from build123d import *

# Parameters (mm, degrees)
SKETCH1_R           = 22.5
SKETCH1_R_2         = 11
BOSS_EXTRUDE1_DEPTH = 11.66


with BuildPart() as part:
    # Sketch1 → Boss-Extrude1 (new body)
    with BuildSketch(Plane(origin=(0, 0, 0), x_dir=(1, 0, 0), z_dir=(0, 1, 0))):
        Circle(SKETCH1_R)
        Circle(SKETCH1_R_2, mode=Mode.SUBTRACT)
    extrude(amount=BOSS_EXTRUDE1_DEPTH)

    # Sketch2 → Revolve1 (revolve)
    with BuildSketch(Plane.XY):
        Polygon((22.5, 11.66), (24.5, 11.66), (24.5, 10.66), (22.5, 10.33), align=None)
        Polygon((22.5, 0.33), (24.5, 0), (24.5, -1), (22.5, -1), (9, -1), (9, 0.33), (9, 4.66), (22.5, 4.66), align=None)
    revolve(axis=Axis((0, 0, 0), (0, 1, 0)))


solid = part.part
Verification items for the finished model (mm, model axes). A direction names the side the tool comes from. Coordinates: 2 decimals unless noted, no trailing zeros. Write each loop counter-clockwise with the first axis right and the second up, starting at its lowest first coordinate (ties: lowest second). Pieces come first, ordered by that corner, then holes. Notation, with made-up numbers: (85, 79.25) - (133, 79.25) arc R21 ccw to (133, 105.25) - close; hole circle Ø10 at (56, 60). An arc over 180 degrees is marked (long way). Answer as a JSON object with one key per item and string values.
(1) Cross-section at D-D on y = 5.5. Record the cut outline in (x, z).
Report:
{"outline": "circle Ø45 at (0, 0); hole circle Ø22 at (0, 0)"}
(2) Cross-section at B-B on z = 0. Record the cut outline in (x, y).
Report:
{"outline": "(-24.5, -1) - (-9, -1) - (-9, 4.66) - (-11, 4.66) - (-11, 11.66) - (-24.5, 11.66) - (-24.5, 10.66) - (-22.5, 10.33) - (-22.5, 0.33) - (-24.5, 0) - close; (9, -1) - (24.5, -1) - (24.5, 0) - (22.5, 0.33) - (22.5, 10.33) - (24.5, 10.66) - (24.5, 11.66) - (11, 11.66) - (11, 4.66) - (9, 4.66) - close"}
(3) Mould release check, pull along X, two halves, no side actions. Record for faces 3 (the flat face through (-2, 4.66, 9)), 4 (the cylindrical face through (10.382, 5.26, 19.961)), 5 (the flat face through (-11, -1, 0)): pulls with the +X half, pulls with the -X half, needs draft (parallel to the pull), parting line crosses it, or undercut.
Report:
{"face 3": "undercut", "face 4": "parting line crosses it", "face 5": "needs draft"}
(4) Tool access check on faces 1 (the cylindrical face through (-2.38, 8.11, 10.74)), 2 (the cylindrical face through (13.17, -0.51, -20.66)). Record the directions out of +Z, -Z, +X, -X, +Y, -Y that give a thin tool (end or side, any length) a straight path to the whole face; none if there is none.
Report:
{"face 1": "+Y", "face 2": "+Y, -Y"}
(5) Cross-section at C-C on y = 2. Record the cut outline in (x, z), plus the area to 3 significant figures.
Report:
{"outline": "circle Ø45 at (0, 0); hole circle Ø18 at (0, 0)", "area": "1,340 mm^2"}
(6) Gauge pin test, flat ends, axial feed: pin 1 Ø1 at (y, z) = (4, -14) entering from -X; pin 2 Ø2 at (x, y) = (3, 9) entering from -Z; pin 3 Ø11 at (x, z) = (0, 0) entering from +Y. Record the tip position at first contact, or that the pin passes through.
Report:
{"pin 1": "x = -18", "pin 2": "z = -22.41", "pin 3": "through"}
(7) Thickness scan on line 1 along Z through (x, y) = (0, 7.75); line 2 along Z through (x, y) = (0, 2.7). Record the ranges inside material, lowest first.
Report:
{"line 1": "-22.5 to -11, 11 to 22.5", "line 2": "-22.5 to -9, 9 to 22.5"}
(8) Cross-section at A-A on x = 0. Record the cut outline in (y, z), plus the area to 3 significant figures.
Report:
{"outline": "(-1, -24.5) - (0, -24.5) - (0.33, -22.5) - (10.33, -22.5) - (10.66, -24.5) - (11.66, -24.5) - (11.66, -11) - (4.66, -11) - (4.66, -9) - (-1, -9) - close; (-1, 9) - (4.66, 9) - (4.66, 11) - (11.66, 11) - (11.66, 24.5) - (10.66, 24.5) - (10.33, 22.5) - (0.33, 22.5) - (0, 24.5) - (-1, 24.5) - close", "area": "323 mm^2"}
